Autodesk Inventor part; units mm, degrees
ref_plane "YZ Plane" through (0, 0, 0) normal (1, 0, 0) x (0, 1, 0)
ref_plane "XZ Plane" through (0, 0, 0) normal (0, 1, 0) x (-1, 0, 0)
ref_plane "XY Plane" through (0, 0, 0) normal (0, 0, 1) x (1, 0, 0)
sketch "Sketch1" plane through (0, 0, 0) normal (0, 1, 0) x (-1, 0, 0)
  circle A0 centre (0, 0) radius 5
  circle A1 centre (0, 0) radius 4.5
  dimension "d0" = 10
  dimension "d1" = 9
extrude "Extrusion1" add sketch "Sketch1" along normal blind 14
chamfer "Chamfer1" distance 0.2 angle 45 1 edges at (5, 14, 0)
chamfer "Chamfer2" distance 0.2 angle 45 1 edges at (5, 0, 0)
properties material "Acetal Resin, Black"
CAD build for the part. Positions are in the model's coordinates, mm. Round coordinates to 2 decimals unless told otherwise and drop trailing zeros. Order: outer loops, then holes, each group sorted by start corner. A loop starts at its lowest first (then second) coordinate and runs counter-clockwise, first axis right, second up.
Q1. Slice it at A-A (z = 0). Write the cut outline in (x, y), and give its area (3 significant figures).
Q2. Slice it at B-B (x = 0). Write the cut outline in (y, z).
Q3. Wall check: L1, parallel to Z at x = 0, y = 11.25; L2, parallel to X at y = 9.25, z = -2.75; L3, parallel to X at y = 7.5, z = -3.5. Give the ranges that are in metal, low to high.
Q4. Slice it at C-C (y = 11). Write the cut outline in (x, z).
Q5. Two-plate mould, pull along Z, no slides. Class faces 1 (the cylindrical face through (1.08, 6.9, 4.88)), 2 (the cylindrical face through (0.59, 6.9, -4.46)): pulls with the +Z half, pulls with the -Z half, needs draft (parallel to the pull), parting line crosses it, or undercut.
Results below:
1. outline: (-5, 0.2) - (-4.8, 0) - (-4.5, 0) - (-4.5, 14) - (-4.8, 14) - (-5, 13.8) - close; (4.5, 0) - (4.8, 0) - (5, 0.2) - (5, 13.8) - (4.8, 14) - (4.5, 14) - close
1. area: 13.9 mm2
2. outline: (0, -4.8) - (0.2, -5) - (13.8, -5) - (14, -4.8) - (14, -4.5) - (0, -4.5) - close; (0, 4.5) - (14, 4.5) - (14, 4.8) - (13.8, 5) - (0.2, 5) - (0, 4.8) - close
3. L1: z = -5 to -4.5, 4.5 to 5
3. L2: x = -4.18 to -3.56, 3.56 to 4.18
3. L3: x = -3.57 to -2.83, 2.83 to 3.57
4. outline: circle Ø10 at (0, 0); hole circle Ø9 at (0, 0)
5. face 1: parting line crosses it
5. face 2: undercut
